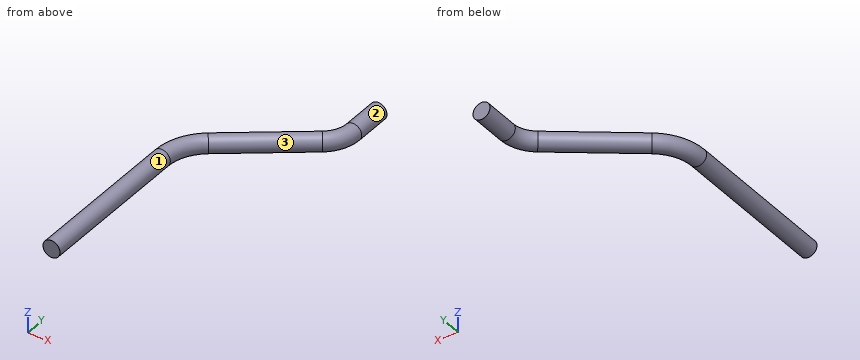
Autodesk Inventor part; units mm, degrees
ref_plane "YZ Plane" through (0, 0, 0) normal (1, 0, 0) x (0, 1, 0)
ref_plane "XZ Plane" through (0, 0, 0) normal (0, 1, 0) x (-1, 0, 0)
ref_plane "XY Plane" through (0, 0, 0) normal (0, 0, 1) x (1, 0, 0)
sketch "Skizze1" plane through (0, 0, 0) normal (0, 0, 1) x (1, 0, 0)
  line L0 (0, 0) -> (0, 30)
  arc A0 (4.5, 39) -> (0, 30) centre (11.25, 30) ccw
  line L1 (4.5, 39) -> (22, 52.125)
  arc A1 (22, 52.125) -> (25, 58.125) centre (17.5, 58.125) ccw
  line L2 (25, 58.125) -> (25, 60)
  line L3 (25, 60) -> (25, 66.5)
  line L4 (0, 0) -> (0, -6.5)
  dimension "d4" = 30
  dimension "d5" = 60
  dimension "d6" = 25
  dimension "d16" = 4.5
  dimension "d17" = 9
  dimension "d18" = 3
  dimension "d19" = 6.5
  dimension "d20" = 6.5
sketch "Skizze2" plane through (0, 0, 0) normal (0, 1, 0) x (-1, 0, 0)
  circle A0 centre (0, 0) radius 2
  dimension "d1" = 4
sweep "Sweeping1" add profiles "Skizze2" path "Skizze1"
equation "\"d20\" = d19"
properties part number "rear iron bar"
CAD build for the part. Positions are in the model's coordinates, mm. Face numbers are marked on the shaded views. A direction names the side the tool comes from. Round coordinates to 2 decimals unless told otherwise and drop trailing zeros. Write each loop counter-clockwise with the first axis right and the second up, starting at its lowest first coordinate (ties: lowest second). Pieces come first, ordered by that corner, then holes.
(1) Drop flat-ended pins along their axis: P1, Ø1.5, axis at y = 48, z = 0.5, coming from the -X side; P2, Ø1, axis at x = 10.5, z = 0.5, coming from the +Y side. Give the stop position or say it passes through.
(2) Slice it at A-A, the plane z = 0. Write the cut outline in (x, y) (3 decimals).
(3) Slice it at B-B, the plane y = 4.5. Write the cut outline in (x, z).
(4) Probe line 1 along X through (y, z) = (12, 0.1); line 2 along Y through (x, z) = (19.75, 1.55); line 3 along X through (y, z) = (49.5, 0.2). List the from-to ranges inside material, lowest first.
(5) 3-axis set-ups, long thin cutter, end or side, ignore diameter. For the marked faces 1, 2 and 3: which of +Z, -Z, +X, -X, +Y, -Y reach the whole face in a straight line?
From the geometry:
1. P1: stops at x = 12.24
1. P2: stops at y = 46.32
2. outline: (-2, -6.5) - (2, -6.5) - (2, 30) arc R9.25 cw to (5.7, 37.4) - (23.2, 50.525) arc R9.5 ccw to (27, 58.125) - (27, 66.5) - (23, 66.5) - (23, 58.125) arc R5.5 cw to (20.8, 53.725) - (3.3, 40.6) arc R13.25 ccw to (-2, 30) - close
3. outline: circle Ø4 at (0, 0)
4. line 1: x = -2 to 2
4. line 2: y = 48.86 to 52.02
4. line 3: x = 15.18 to 21.82
5. face 1: -Y
5. face 2: +Y
5. face 3: none
